Check sheet for the drawn part. Datum: minimum x, y, z corner. Units: mm. A direction names the side the tool comes from. Round coordinates to 2 decimals unless told otherwise and drop trailing zeros. Loops run counter-clockwise (first coordinate to the right, second up) from the corner with the lowest first, then second, coordinate; pieces in that order, holes last.
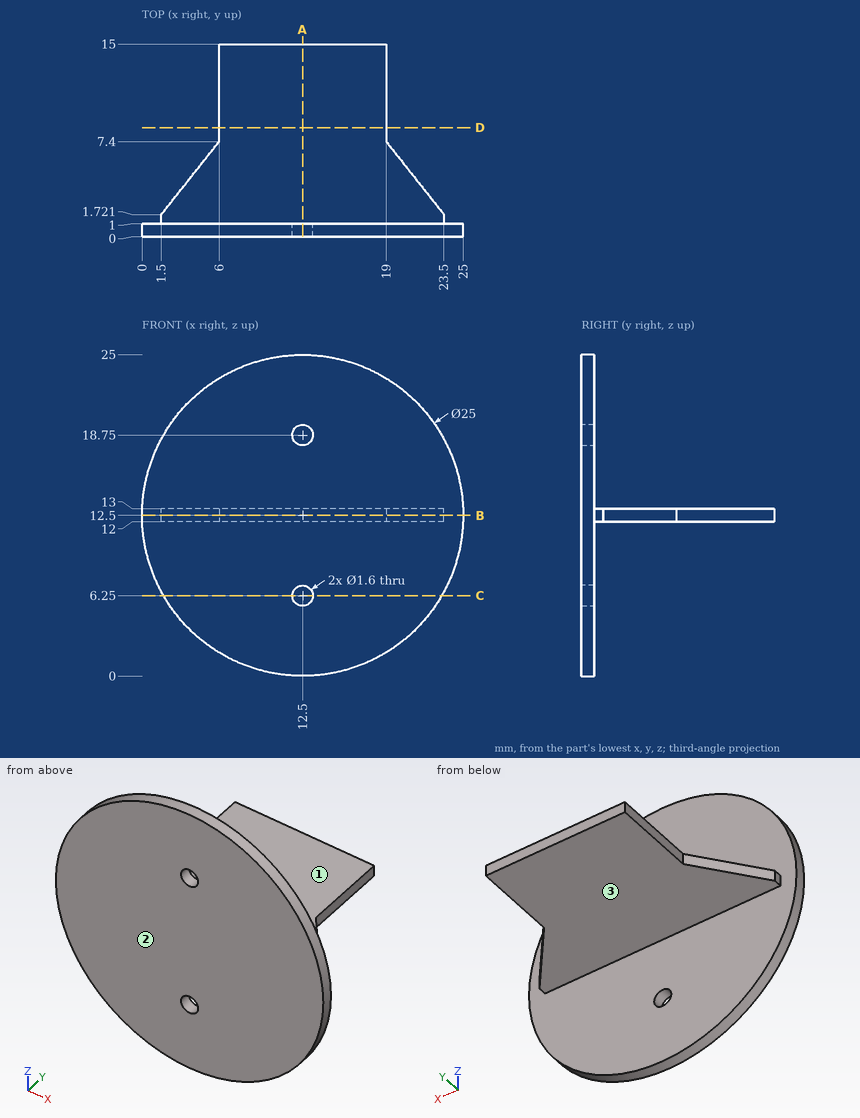
1. Scan lines: L1, parallel to Y at x = 6, z = 15.75; L2, parallel to Z at x = 6.25, y = 7; L3, parallel to X at y = 0.5, z = 6.25 (1 decimal). Record each from-to range of solid material in increasing order.
2. Section check A-A (x = 12.5). Enter the section's corners in (y, z), then the cut area to 3 significant figures.
3. Gauge pin test, flat ends, axial feed: P1, Ø1.5, axis at x = 7.5, y = 9, coming from the +Z side; P2, Ø7.5, axis at x = 10.5, z = 18, coming from the +Y side; P3, Ø1.1, axis at y = 12.5, z = 12.5, coming from the +X side. Record the tip position at first contact, or that the pin passes through.
4. Section check C-C (z = 6.25). Enter the section's corners in (x, y) (1 decimal).
5. Tool access check on the marked faces 1, 2 and 3. Record the directions out of +Z, -Z, +X, -X, +Y, -Y that give a thin tool (end or side, any length) a straight path to the whole face; none if there is none.
6. Section check B-B (z = 12.5). Enter the section's corners in (x, y).
7. Section check D-D (y = 8.5). Enter the section's corners in (x, z), then the cut area to 3 significant figures.
Taken from the geometry:
1. L1: y = 0 to 1
1. L2: z = 12 to 13
1. L3: x = 1.7 to 11.7, 13.3 to 23.3
2. outline: (0, 0) - (1, 0) - (1, 5.45) - (0, 5.45) - close; (0, 7.05) - (1, 7.05) - (1, 12) - (15, 12) - (15, 13) - (1, 13) - (1, 17.95) - (0, 17.95) - close; (0, 19.55) - (1, 19.55) - (1, 25) - (0, 25) - close
2. area: 35.8 mm2
3. P1: stops at z = 13
3. P2: stops at y = 1
3. P3: stops at x = 19
4. outline: (1.7, 0) - (11.7, 0) - (11.7, 1) - (1.7, 1) - close; (13.3, 0) - (23.3, 0) - (23.3, 1) - (13.3, 1) - close
5. face 1: +Z, +X, -X, +Y
5. face 2: +Z, -Z, +X, -X, -Y
5. face 3: -Z, +X, -X, +Y
6. outline: (0, 0) - (25, 0) - (25, 1) - (23.5, 1) - (23.5, 1.72) - (19, 7.4) - (19, 15) - (6, 15) - (6, 7.4) - (1.5, 1.72) - (1.5, 1) - (0, 1) - close
7. outline: (6, 12) - (19, 12) - (19, 13) - (6, 13) - close
7. area: 13.0 mm2
